Design review of the part built by this model. Coordinates are the model's own, in mm. Face numbers are marked on the shaded views. A direction names the side the tool comes from. Give positions to 0.01 mm unless a question says otherwise; leave off trailing zeros. Order: outer loops, then holes, each group sorted by start corner. A loop starts at its lowest first (then second) coordinate and runs counter-clockwise, first axis right, second up. Notation, with made-up numbers: (-0.75, 35.5) -> (11.25, 35.5) arc R11 ccw to (11.25, 51.5) -> close; hole circle Ø3 at (83, -23). An arc over 180 degrees is marked (long way). Answer in a Markdown table with one row per item. Add a question column.
```python
from build123d import *

# Parameters (mm, degrees)
SKETCH_1_R               = 1.265
EXTRUDE_1_DEPTH          = 10
SKETCH_2_R               = 2.75
SKETCH_2_R_2             = 1.265
EXTRUDE_2_DEPTH          = 1.2
SKETCH_3_R               = 10.210079725
SKETCH_3_R_2             = 7.3
CUT_EXTRUDE_2_DEPTH      = 16.316956182
FILLET_1_R               = 0.5
PATTERN_CIRCULAR_2_DEPTH = 10


# Read off the part's stored shape, not the designer's step: Круговой массив2
with BuildPart() as part:
    # Эскиз1 → Бобышка-Вытянуть1 (new body)
    with BuildSketch(Plane.XY):
        with BuildLine():
            ThreePointArc((-3.148803906, 3.471068454), (-4.227852242, 4.566214035), (-5.743712894, 4.822837566))
            ThreePointArc((-5.743712894, 4.822837566), (-5.841480421, 4.703945843), (-5.936787387, 4.583072716))
            ThreePointArc((-5.936787387, 4.583072716), (-5.362797198, 3.156810321), (-4.062728379, 2.336133637))
            ThreePointArc((-4.062728379, 2.336133637), (-4.379801209, 1.667520202), (-4.587678719, 0.95733287))
            ThreePointArc((-4.587678719, 0.95733287), (-6.104357582, 1.209075557), (-7.481554138, 0.525687819))
            ThreePointArc((-7.481554138, 0.525687819), (-7.490766927, 0.372036085), (-7.496824441, 0.218227641))
            ThreePointArc((-7.496824441, 0.218227641), (-6.194120622, -0.598259906), (-4.659961201, -0.498040012))
            ThreePointArc((-4.659961201, -0.498040012), (-4.523477392, -1.225330377), (-4.274216191, -1.922071332))
            ThreePointArc((-4.274216191, -1.922071332), (-5.649205805, -2.609888688), (-6.361695989, -3.972256807))
            ThreePointArc((-6.361695989, -3.972256807), (-6.278835069, -4.101978813), (-6.193329365, -4.229972975))
            ThreePointArc((-6.193329365, -4.229972975), (-4.659500498, -4.124815183), (-3.477247231, -3.141979304))
            ThreePointArc((-3.477247231, -3.141979304), (-2.939338959, -3.650146399), (-2.328148353, -4.067309614))
            ThreePointArc((-2.328148353, -4.067309614), (-3.03624942, -5.431964161), (-2.811886199, -6.952934345))
            ThreePointArc((-2.811886199, -6.952934345), (-2.668601624, -7.009177225), (-2.524192976, -7.062467686))
            ThreePointArc((-2.524192976, -7.062467686), (-1.345109555, -6.075831258), (-0.966343005, -4.585789294))
            ThreePointArc((-0.966343005, -4.585789294), (-0.232472948, -4.68073056), (0.507193024, -4.658973866))
            ThreePointArc((0.507193024, -4.658973866), (0.736451045, -6.179213951), (1.811968547, -7.277827285))
            ThreePointArc((1.811968547, -7.277827285), (1.960946938, -7.239108171), (2.109099336, -7.197339786))
            ThreePointArc((2.109099336, -7.197339786), (2.483067519, -5.706086302), (1.913671403, -4.277983638))
            ThreePointArc((1.913671403, -4.277983638), (2.563189827, -3.92343474), (3.148803906, -3.471068454))
            ThreePointArc((3.148803906, -3.471068454), (4.227852242, -4.566214035), (5.743712894, -4.822837566))
            ThreePointArc((5.743712894, -4.822837566), (5.841480421, -4.703945843), (5.936787387, -4.583072716))
            ThreePointArc((5.936787387, -4.583072716), (5.362797198, -3.156810321), (4.062728379, -2.336133637))
            ThreePointArc((4.062728379, -2.336133637), (4.379801209, -1.667520202), (4.587678719, -0.95733287))
            ThreePointArc((4.587678719, -0.95733287), (6.104357582, -1.209075557), (7.481554138, -0.525687819))
            ThreePointArc((7.481554138, -0.525687819), (7.490766927, -0.372036085), (7.496824441, -0.218227641))
            ThreePointArc((7.496824441, -0.218227641), (6.194120622, 0.598259906), (4.659961201, 0.498040012))
            ThreePointArc((4.659961201, 0.498040012), (4.523477392, 1.225330377), (4.274216191, 1.922071332))
            ThreePointArc((4.274216191, 1.922071332), (5.649205805, 2.609888688), (6.361695989, 3.972256807))
            ThreePointArc((6.361695989, 3.972256807), (6.278835069, 4.101978813), (6.193329365, 4.229972975))
            ThreePointArc((6.193329365, 4.229972975), (4.659500498, 4.124815183), (3.477247231, 3.141979304))
            ThreePointArc((3.477247231, 3.141979304), (2.939338959, 3.650146399), (2.328148353, 4.067309614))
            ThreePointArc((2.328148353, 4.067309614), (3.03624942, 5.431964161), (2.811886199, 6.952934345))
            ThreePointArc((2.811886199, 6.952934345), (2.668601624, 7.009177225), (2.524192976, 7.062467686))
            ThreePointArc((2.524192976, 7.062467686), (1.345109555, 6.075831258), (0.966343005, 4.585789294))
            ThreePointArc((0.966343005, 4.585789294), (0.232472948, 4.68073056), (-0.507193024, 4.658973866))
            ThreePointArc((-0.507193024, 4.658973866), (-0.736451045, 6.179213951), (-1.811968547, 7.277827285))
            ThreePointArc((-1.811968547, 7.277827285), (-1.960946938, 7.239108171), (-2.109099336, 7.197339786))
            ThreePointArc((-2.109099336, 7.197339786), (-2.483067519, 5.706086302), (-1.913671403, 4.277983638))
            ThreePointArc((-1.913671403, 4.277983638), (-2.563189827, 3.92343474), (-3.148803906, 3.471068454))
        make_face()
        Circle(SKETCH_1_R, mode=Mode.SUBTRACT)
    extrude(amount=EXTRUDE_1_DEPTH)

    # Эскиз2 → Бобышка-Вытянуть2 (add)
    with BuildSketch(Plane.XY.offset(10)):
        Circle(SKETCH_2_R)
        Circle(SKETCH_2_R_2, mode=Mode.SUBTRACT)
    extrude(amount=EXTRUDE_2_DEPTH)

    # Эскиз3 → Вырез-Вытянуть2 (cut, through all)
    with BuildSketch(Plane(origin=(0, 0, 0), x_dir=(-1, 0, 0), z_dir=(0, 0, -1))):
        Circle(SKETCH_3_R)
        Circle(SKETCH_3_R_2, mode=Mode.SUBTRACT)
    extrude(amount=-CUT_EXTRUDE_2_DEPTH, mode=Mode.SUBTRACT)

    # Скругление1
    fillet_1_edges = [part.edges().sort_by_distance(p)[0] for p in [
        (-2.246892365, 6.945608303, 5),
        (-1.565958675, 7.13006125, 5),
    ]]
    fillet(fillet_1_edges, radius=FILLET_1_R)

    # Круговой массив2 outline → Круговой массив2 (cut)
    with BuildSketch(Plane.XY):
        with BuildLine():
            ThreePointArc((-5.838293306, 4.042408612), (-5.850561559, 4.278183981), (-5.753278974, 4.493304024))
            ThreePointArc((-5.753278974, 4.493304024), (-5.827604273, 4.396479095), (-5.900300237, 4.298424958))
            ThreePointArc((-5.900300237, 4.298424958), (-5.872671085, 4.169599529), (-5.838293306, 4.042408612))
        make_face()
        with BuildLine():
            ThreePointArc((-5.457832031, 4.847893307), (-5.538127486, 4.755958783), (-5.61687454, 4.662694543))
            ThreePointArc((-5.61687454, 4.662694543), (-5.427449488, 4.803615386), (-5.19448163, 4.841910441))
            ThreePointArc((-5.19448163, 4.841910441), (-5.326077976, 4.84837285), (-5.457832031, 4.847893307))
        make_face()
        with BuildLine():
            ThreePointArc((-7.099346669, -0.161285439), (-7.247857179, 0.022249743), (-7.295598302, 0.253466783))
            ThreePointArc((-7.295598302, 0.253466783), (-7.298816468, 0.131446456), (-7.299993962, 0.009389377))
            ThreePointArc((-7.299993962, 0.009389377), (-7.201919821, -0.078592576), (-7.099346669, -0.161285439))
        make_face()
        with BuildLine():
            ThreePointArc((-7.264999056, 0.713994895), (-7.275921686, 0.592421818), (-7.284810046, 0.470683106))
            ThreePointArc((-7.284810046, 0.470683106), (-7.214393154, 0.696031715), (-7.048427465, 0.863948137))
            ThreePointArc((-7.048427465, 0.863948137), (-7.158689654, 0.791825944), (-7.264999056, 0.713994895))
        make_face()
        with BuildLine():
            ThreePointArc((-5.648690902, -4.303373934), (-5.876717701, -4.24218314), (-6.051247048, -4.083186154))
            ThreePointArc((-6.051247048, -4.083186154), (-5.982128849, -4.183794263), (-5.911338111, -4.283232627))
            ThreePointArc((-5.911338111, -4.283232627), (-5.78027997, -4.296764989), (-5.648690902, -4.303373934))
        make_face()
        with BuildLine():
            ThreePointArc((-6.29718337, -3.692625299), (-6.234561102, -3.797400146), (-6.170195716, -3.90111328))
            ThreePointArc((-6.170195716, -3.90111328), (-6.245683843, -3.677412414), (-6.210113576, -3.444012991))
            ThreePointArc((-6.210113576, -3.444012991), (-6.2569252, -3.567171559), (-6.29718337, -3.692625299))
        make_face()
        with BuildLine():
            ThreePointArc((-2.040427202, -6.801719852), (-2.260871804, -6.88624625), (-2.495525095, -6.860200762))
            ThreePointArc((-2.495525095, -6.860200762), (-2.380471335, -6.900967774), (-2.264752021, -6.939805349))
            ThreePointArc((-2.264752021, -6.939805349), (-2.150769635, -6.873719217), (-2.040427202, -6.801719852))
        make_face()
        with BuildLine():
            ThreePointArc((-2.92405767, -6.688788137), (-2.811810081, -6.736744322), (-2.69877634, -6.782816986))
            ThreePointArc((-2.69877634, -6.782816986), (-2.891335587, -6.646209992), (-2.999747375, -6.436478214))
            ThreePointArc((-2.999747375, -6.436478214), (-2.965227985, -6.563630771), (-2.92405767, -6.688788137))
        make_face()
        with BuildLine():
            ThreePointArc((2.347210337, -6.702039969), (2.218550278, -6.899997348), (2.013402624, -7.016851849))
            ThreePointArc((2.013402624, -7.016851849), (2.130445319, -6.982206151), (2.246892365, -6.945608303))
            ThreePointArc((2.246892365, -6.945608303), (2.300261598, -6.825146334), (2.347210337, -6.702039969))
        make_face()
        with BuildLine():
            ThreePointArc((1.565958675, -7.13006125), (1.684956821, -7.102881142), (1.80348387, -7.073715143))
            ThreePointArc((1.80348387, -7.073715143), (1.56740459, -7.076381249), (1.356420365, -6.970427527))
            ThreePointArc((1.356420365, -6.970427527), (1.459085537, -7.053006118), (1.565958675, -7.13006125))
        make_face()
        with BuildLine():
            ThreePointArc((5.838293306, -4.042408612), (5.850561559, -4.278183981), (5.753278974, -4.493304024))
            ThreePointArc((5.753278974, -4.493304024), (5.827604273, -4.396479095), (5.900300237, -4.298424958))
            ThreePointArc((5.900300237, -4.298424958), (5.872671085, -4.169599529), (5.838293306, -4.042408612))
        make_face()
        with BuildLine():
            ThreePointArc((5.457832031, -4.847893307), (5.538127486, -4.755958783), (5.61687454, -4.662694543))
            ThreePointArc((5.61687454, -4.662694543), (5.427449488, -4.803615386), (5.19448163, -4.841910441))
            ThreePointArc((5.19448163, -4.841910441), (5.326077976, -4.84837285), (5.457832031, -4.847893307))
        make_face()
        with BuildLine():
            ThreePointArc((7.099346669, 0.161285439), (7.247857179, -0.022249743), (7.295598302, -0.253466783))
            ThreePointArc((7.295598302, -0.253466783), (7.298816468, -0.131446456), (7.299993962, -0.009389377))
            ThreePointArc((7.299993962, -0.009389377), (7.201919821, 0.078592576), (7.099346669, 0.161285439))
        make_face()
        with BuildLine():
            ThreePointArc((7.264999056, -0.713994895), (7.275921686, -0.592421818), (7.284810046, -0.470683106))
            ThreePointArc((7.284810046, -0.470683106), (7.214393154, -0.696031715), (7.048427465, -0.863948137))
            ThreePointArc((7.048427465, -0.863948137), (7.158689654, -0.791825944), (7.264999056, -0.713994895))
        make_face()
        with BuildLine():
            ThreePointArc((5.648690902, 4.303373934), (5.876717701, 4.24218314), (6.051247048, 4.083186154))
            ThreePointArc((6.051247048, 4.083186154), (5.982128849, 4.183794263), (5.911338111, 4.283232627))
            ThreePointArc((5.911338111, 4.283232627), (5.78027997, 4.296764989), (5.648690902, 4.303373934))
        make_face()
        with BuildLine():
            ThreePointArc((6.29718337, 3.692625299), (6.234561102, 3.797400146), (6.170195716, 3.90111328))
            ThreePointArc((6.170195716, 3.90111328), (6.245683843, 3.677412414), (6.210113576, 3.444012991))
            ThreePointArc((6.210113576, 3.444012991), (6.2569252, 3.567171559), (6.29718337, 3.692625299))
        make_face()
        with BuildLine():
            ThreePointArc((2.040427202, 6.801719852), (2.260871804, 6.88624625), (2.495525095, 6.860200762))
            ThreePointArc((2.495525095, 6.860200762), (2.380471335, 6.900967774), (2.264752021, 6.939805349))
            ThreePointArc((2.264752021, 6.939805349), (2.150769635, 6.873719217), (2.040427202, 6.801719852))
        make_face()
        with BuildLine():
            ThreePointArc((2.92405767, 6.688788137), (2.811810081, 6.736744322), (2.69877634, 6.782816986))
            ThreePointArc((2.69877634, 6.782816986), (2.891335587, 6.646209992), (2.999747375, 6.436478214))
            ThreePointArc((2.999747375, 6.436478214), (2.965227985, 6.563630771), (2.92405767, 6.688788137))
        make_face()
    extrude(amount=PATTERN_CIRCULAR_2_DEPTH, mode=Mode.SUBTRACT)


solid = part.part
```
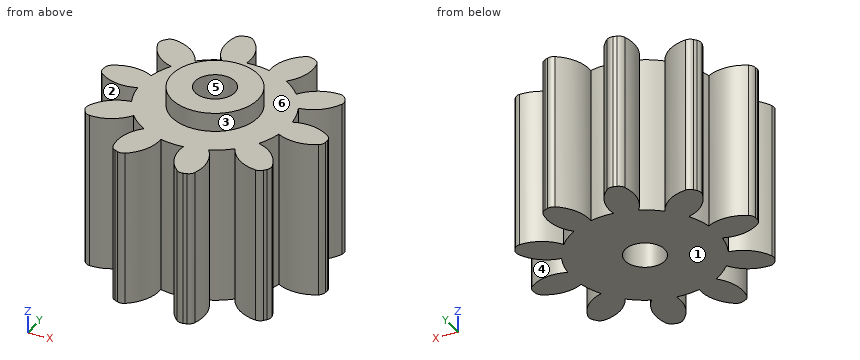
1) Machinability: for the marked faces 5 and 6, which of the approach directions +Z, -Z, +X, -X, +Y, -Y give a long, thin tool a straight path to every point of the face, cutting with its end or side? Answer none if there is none.
2) Clearance check with flat-ended pins moving along their axes: P1, Ø1.5, axis at x = 0.5, z = 10, coming from the +Y side; P2, Ø6, axis at x = -2, y = -5.5, coming from the +Z side; P3, Ø2, axis at x = 1, z = 2, coming from the +Y side. State where each tip first meets the part, or that it passes through.
3) Add section B-B, the plane y = -5.75. Write out the cut boundary in (x, z), and give its area (3 significant figures).
4) Mouldability with a two-part tool opening along Y and no side actions: class the marked faces 1, 2, 3 and 4 as +Y half, -Y half, draft (parallel to the pull), parting line (faces both ways), or undercut.
5) For L1, parallel to Y at x = 0, z = 7.75 (1 decimal); L2, parallel to Z at x = -1, y = -4.75; L3, parallel to X at y = -5.5, z = 5.5, list the stretches that pass through material, from the lowest coordinate up.
Verdict:
| question | item | result |
|---|---|---|
| 1 | face 5 | +Z, -Z |
| 1 | face 6 | +Z |
| 2 | P1 | stops at y = 5.91 |
| 2 | P2 | stops at z = 10 |
| 2 | P3 | stops at y = 6.77 |
| 3 | outline | (-3.07, 0) -> (-1.17, 0) -> (-1.17, 10) -> (-3.07, 10) -> close; (0.57, 0) -> (2.49, 0) -> (2.49, 10) -> (0.57, 10) -> close |
| 3 | area | 38.1 mm2 |
| 4 | face 1 | draft |
| 4 | face 2 | undercut |
| 4 | face 3 | parting line |
| 4 | face 4 | undercut |
| 5 | L1 | y = -4.7 to -1.3, 1.3 to 4.7 |
| 5 | L2 | z = 0 to 10 |
| 5 | L3 | x = -3.05 to -1.08, 0.51 to 2.46 |
